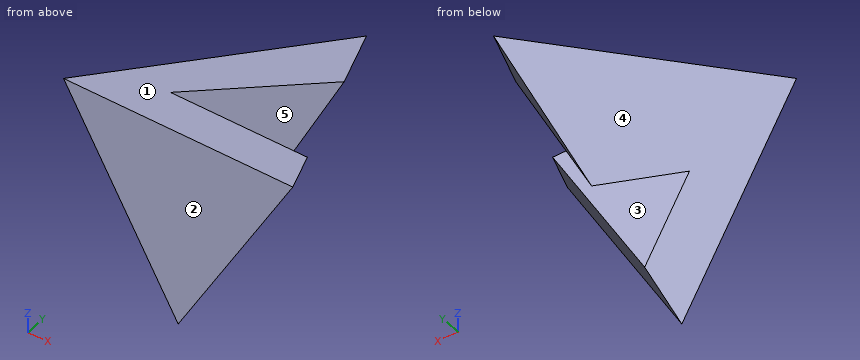
```python
from build123d import *

# Parameters (mm, degrees)
CUT_EXTRUDE_2_DEPTH = 38


with BuildPart() as part:
    # 草图1 → 放样3 section 0
    with BuildSketch(Plane(origin=(0, 0, 0), x_dir=(1, 0, 0), z_dir=(0, 1, 0)), mode=Mode.PRIVATE) as loft_3_s0:
        Polygon((0, 39.837168574), (-34.5, -19.918584287), (34.5, -19.918584287), align=None)
    loft([Vertex(0, 76, 0), loft_3_s0.sketch])

    # 草图11 → 切除-拉伸2 (cut, symmetric)
    with BuildSketch(Plane.XY):
        Polygon((10.440789474, 53), (27.690789474, 15), (-13.5, 15), align=None)
    extrude(amount=CUT_EXTRUDE_2_DEPTH, both=True, mode=Mode.SUBTRACT)


solid = part.part
```
Here's how the part is built. I have some questions about the finished solid (model axes, mm). Face numbers are marked on the shaded views. A direction names the side the tool comes from. Give positions to 0.01 mm unless a question says otherwise; leave off trailing zeros. Loops run counter-clockwise (first coordinate to the right, second up) from the corner with the lowest first, then second, coordinate; pieces in that order, holes last. Notation, with made-up numbers: M 76.5,-23 L 117.5,-23 A6 cw 117.5,-15 Z; hole C -5,10 d1. An arc over 180 degrees is marked long. Put each result on its own line as item: value. Start each with the question number.
(1) I want a section at A-A on z = -12. Please give me the cut outline in (x, y), then the cut area to 3 significant figures.
(2) Will these pins go through, and if not, where does the flat tip stop? pin 1 Ø3 at (x, y) = (-15.5, 10) entering from +Z; pin 2 Ø1 at (y, z) = (41.5, -4) entering from +X; pin 3 Ø2 at (x, z) = (8.5, -14) entering from +Y.
(3) I need wall thicknesses on line 1 along X through (y, z) = (8, 5.5); line 2 along Z through (x, y) = (-10, 21.5); line 3 along Z through (x, y) = (11, 13). Which ranges of each line are inside material? Lowest first, please. Write a range as [from, to].
(4) If we mould it in two halves opening along Y, with no side actions, what happens to the marked faces 1, 2 and 3? For each: +Y half, -Y half, draft (parallel to the pull), parting line (faces both ways), or undercut.
(5) For the marked faces 4 and 5, which set-ups out of +Z, -Z, +X, -X, +Y, -Y let a thin tool reach every point of the face, with its end or its side?
(6) I want a section at B-B on x = -6. Please give me the cut outline in (y, z), then the cut area to 3 significant figures.
(7) I want a section at C-C on z = -1.5. Please give me the cut outline in (x, y).
(8) I want a section at D-D on y = 23. Please give me the cut outline in (x, z), then the cut area to 3 significant figures.
Answer block:
1. outline: M -16.07,0 L 16.07,0 L 11.53,15 L -11.53,15 Z; M -9.71,21.01 L 3.41,41.84 L 0,53.11 Z
1. area: 524 mm^2
2. pin 1: z = 17.69
2. pin 2: x = 3.51
2. pin 3: y = 15
3. line 1: [-23.75, 23.75]
3. line 2: [-11.25, 14.28]
3. line 3: [-13.97, 16.51]
4. face 1: +Y half
4. face 2: -Y half
4. face 3: undercut
5. face 4: -Z, -X, +Y
5. face 5: +Z, -Z, +X
6. outline: M 0,-29.44 L 15,-21.58 L 15,15.99 L 0,19.92 Z; M 26.9,-15.34 L 62.78,3.46 L 26.9,12.87 Z
6. area: 1,160 mm^2
7. outline: M -22.13,0 L 22.13,0 L 17.59,15 L -13.5,15 L 7.5,48.34 L 0,73.14 Z
8. outline: M -24.06,13.89 L -8.46,-13.13 L -8.46,13.89 Z
8. area: 211 mm^2
